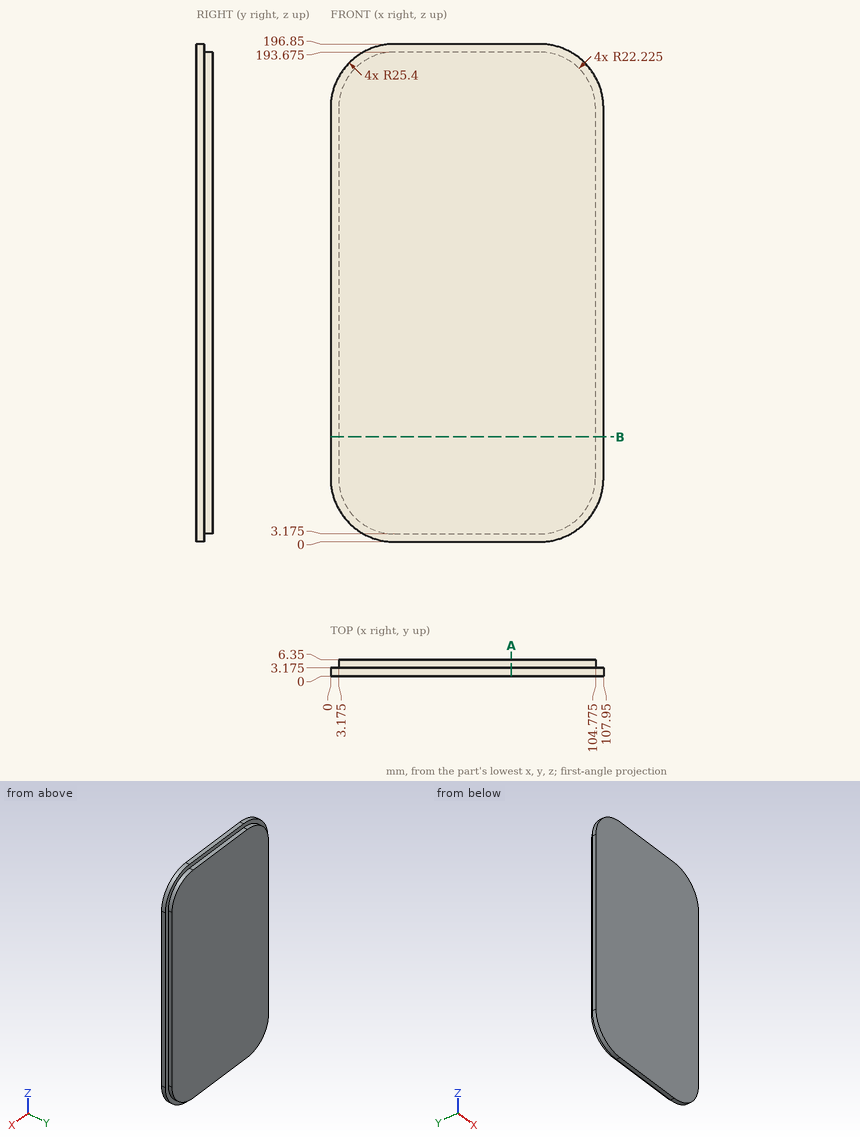
Input: dimensioned drawing with shaded views. Units: mm. Origin: part minimum x, y, z. Give positions to 0.01 mm unless a question says otherwise; leave off trailing zeros. Loops run counter-clockwise (first coordinate to the right, second up) from the corner with the lowest first, then second, coordinate; pieces in that order, holes last. Notation, with made-up numbers: (53.5, 33) - (61.5, 33) arc R26 cw to (61.5, 71) - close; hole circle Ø3 at (-39.5, 84.5). An arc over 180 degrees is marked (long way). Answer as CSV lines item,"result". Start each with the question number.
(1) Pin query (flat end, axial travel): P1, Ø3.5, axis at x = 42.5, y = 5, coming from the -Z side (3 decimals); P2, Ø1.5, axis at x = 71.5, y = 2, coming from the -Z side; P3, Ø2, axis at x = 49.5, y = 4.5, coming from the +Z side (3 decimals); P4, Ø2, axis at y = 4.5, z = 117, coming from the -X side (3 decimals). Return the tip coordinate at first contact, or that it passes through.
(2) Section query A-A (x = 71.5). Output: boundary loops of the cut face in (y, z) (3 decimals), and give its area (3 significant figures).
(3) Ray query, line 1 along Z through (x, y) = (63, 6) (3 decimals); line 2 along X through (y, z) = (4.5, 140.5) (3 decimals); line 3 along Z through (x, y) = (97, 6). Return the intervals inside material, ascending. Write a range as [from, to].
(4) Section query B-B (z = 41.5). Output: boundary loops of the cut face in (x, y) (3 decimals), and give its area (3 significant figures).
Worked answers:
1,P1,"stops at z = 3.175"
1,P2,"stops at z = 0"
1,P3,"stops at z = 193.675"
1,P4,"stops at x = 3.175"
2,outline,"(0, 0) - (3.175, 0) - (3.175, 3.175) - (6.35, 3.175) - (6.35, 193.675) - (3.175, 193.675) - (3.175, 196.85) - (0, 196.85) - close"
2,area,"1,230 mm^2"
3,line 1,"z = [3.175, 193.675]"
3,line 2,"x = [3.175, 104.775]"
3,line 3,"z = [8.51, 188.34]"
4,outline,"(0, 0) - (107.95, 0) - (107.95, 3.175) - (104.775, 3.175) - (104.775, 6.35) - (3.175, 6.35) - (3.175, 3.175) - (0, 3.175) - close"
4,area,"665 mm^2"
